```python
from build123d import *

# Parameters (mm, degrees)
F3_D     = 9.525
F3_DEPTH = 9.525
F3_TIP   = 2.8615986981
F4_R     = 1.5875
F5_DEPTH = 48.27


with BuildPart() as f1:
    # F0 (on Front) → F1 (revolve)
    with BuildSketch(Plane.XZ):
        Polygon((0, -44.6369265472), (0, 0), (-9.1277007014, 0), (-9.1277007014, -14.6898925304), (-14.9883243068, -14.6898925304), (-19.7362518723, -26.5907669723), align=None)
    revolve(axis=Axis((0, 0, -22.3184632736), (0, 0, -1)))

    # F3
    with Locations(Plane.XY):
        with Locations((0, 0)):
            Hole(F3_D / 2, depth=F3_DEPTH)
            with Locations((0, 0, -(F3_DEPTH + F3_TIP / 2))):  # 118° drill point
                Cone(0, F3_D / 2, F3_TIP, mode=Mode.SUBTRACT)

    # F4 (on Top) → F5 (cut)
    with BuildSketch(Plane.XY):
        Circle(F4_R)
    extrude(amount=-F5_DEPTH, mode=Mode.SUBTRACT)


solid = f1.part
```
Input: part model. Units: mm. Frame: model coordinates. A direction names the side the tool comes from. Give positions to 0.01 mm unless a question says otherwise; leave off trailing zeros. Order: outer loops, then holes, each group sorted by start corner. A loop starts at its lowest first (then second) coordinate and runs counter-clockwise, first axis right, second up. Notation, with made-up numbers: M 32.5,21 L 90.5,21 A31 cw 90.5,57 Z; hole C 16.5,-3.75 d9. An arc over 180 degrees is marked long. One line per question, with ' | ' between items.
1) Access query for faces 4 (the face through (3.78, -2.9, -4.83)), 5 (the face through (0.972, -4.379, -40.536)). Directions: +Z, -Z, +X, -X, +Y, -Y. A direction counts if a zero-diameter tool reaches every point of the face in a straight line with its end or side. Return the directions, or none.
Filled in:
face 4: +Z | face 5: -Z
2) Section A-A on x = 0. Output: boundary loops of the cut face in (y, z) (1 decimal), and give its area (3 significant figures).
Filled in:
outline: M -19.7,-26.6 L -1.6,-43.2 L -1.6,-11.4 L -4.8,-9.5 L -4.8,0 L -9.1,0 L -9.1,-14.7 L -15,-14.7 Z; M 1.6,-43.2 L 19.7,-26.6 L 15,-14.7 L 9.1,-14.7 L 9.1,0 L 4.8,0 L 4.8,-9.5 L 1.6,-11.4 Z | area: 832 mm2
3) Section C-C on z = -3. Output: boundary loops of the cut face in (x, y) (1 decimal).
Filled in:
outline: C 0,0 d18.3; hole C 0,0 d9.5
4) Ray query, L1, parallel to X at y = -1, z = -13.5; L2, parallel to X at y = 0, z = -22; L3, parallel to Y at x = 0, z = -36. Return the intervals inside material, ascending.
Filled in:
L1: x = -9.07 to -1.23, 1.23 to 9.07 | L2: x = -17.9 to -1.59, 1.59 to 17.9 | L3: y = -9.45 to -1.59, 1.59 to 9.45
5) Draft query along Y for faces 1 (the face through (-1.26, -0.966, -27.087)), 2 (the face through (6.5, 6.9, -14.69)), 3 (the face through (1.98, -8.91, -7.45)). Return one class per face: pulls with the +Y half, pulls with the -Y half, needs draft (parallel to the pull), parting line crosses it, or undercut.
Filled in:
face 1: undercut | face 2: needs draft | face 3: parting line crosses it
6) Section D-D on z = -20.5. Output: boundary loops of the cut face in (x, y) (1 decimal), and give its area (3 significant figures).
Filled in:
outline: C 0,0 d34.6; hole C 0,0 d3.2 | area: 933 mm2
7) Contact query for flat-ended pins moving along their axis: P1, Ø12.5, axis at x = 0, y = 0, coming from the +Z side; P2, Ø2, axis at y = 15.5, z = -21.5, coming from the +X side; P3, Ø1, axis at x = -11, z = -17, coming from the +Y side; P4, Ø10, axis at x = -6, y = 13.5, coming from the +Z side. Output: stop coordinate, or through.
Filled in:
P1: stops at z = 0 | P2: stops at x = 10.32 | P3: stops at y = 12.03 | P4: stops at z = -14.69
